For this review, take the finished solid that the model builds, in its own axes (mm). Coordinates: 2 decimals unless noted, no trailing zeros. Write each loop counter-clockwise with the first axis right and the second up, starting at its lowest first coordinate (ties: lowest second). Pieces come first, ordered by that corner, then holes. Notation, with made-up numbers: (60, 67) -> (80, 67) arc R37 ccw to (80, 104) -> close; hole circle Ø3 at (81.25, 66.25). An arc over 180 degrees is marked (long way). Put each result on its own line as item: value. Start each with the question number.
Item 1: To check wall thickness, follow L1, parallel to Z at x = -25, y = 3.2; L2, parallel to Z at x = -43.5, y = 0.3; L3, parallel to X at y = 1.55, z = 52. State the ranges of each line that lie inside material, in increasing order.
Item 2: Consider section C-C on x = -75. Give the boundary of the cut face in (y, z), and give its area (3 significant figures).
Item 3: Consider section B-B on z = -6. Give the boundary of the cut face in (x, y), and give its area (3 significant figures).
Item 4: Insertion check: P1, Ø10, axis at x = 44, z = 39.5, coming from the -Y side. The pin has a flat end and moves straight along its axis. Give the tip position at first contact, or say it passes through.
Item 5: The part is to be moulded in two halves that separate along Z. For faces 1 (the flat face through (-31, 0, -1)), 2 (the cylindrical face through (126.99, 2.03, -66.15)), 3 (the cylindrical face through (126.99, 2.03, 66.15)), 4 (the cylindrical face through (7.21, 2.03, 22.89)), say which applies: +Z half, -Z half, draft (parallel to the pull), parting line (faces both ways), or undercut.
Item 6: Consider section D-D on z = -20.5. Give the boundary of the cut face in (x, y), and give its area (3 significant figures).
Item 7: Consider section A-A on x = 0. Give the boundary of the cut face in (y, z), and give its area (3 significant figures).
```python
from build123d import *

# Parameters (mm, degrees)
SKETCH_1_W          = 260
SKETCH_1_H          = 138
SKETCH_1_R          = 1.35
EXTRUDE_1_DEPTH     = 4
SKETCH_3_R          = 24
SKETCH_3_R_2        = 1.65
CUT_EXTRUDE_1_DEPTH = 4
CUT_EXTRUDE_3_DEPTH = 4
FILLET_1_R          = 10


with BuildPart() as part:
    # 草图1 → 凸台-拉伸1 (new body)
    with BuildSketch(Plane(origin=(0, 0, 0), x_dir=(1, 0, 0), z_dir=(0, 1, 0))):
        Rectangle(SKETCH_1_W, SKETCH_1_H)
        with Locations(Location((-122, 64, 0), (0, 0, 270))):
            Circle(SKETCH_1_R, mode=Mode.SUBTRACT)
        with Locations(Location((122, 64, 0), (0, 0, 90))):
            Circle(SKETCH_1_R, mode=Mode.SUBTRACT)
        with Locations(Location((122, -64, 0), (0, 0, 270))):
            Circle(SKETCH_1_R, mode=Mode.SUBTRACT)
        with Locations(Location((-122, -64, 0), (0, 0, 90))):
            Circle(SKETCH_1_R, mode=Mode.SUBTRACT)
    extrude(amount=EXTRUDE_1_DEPTH)

    # 草图3 → 切除-拉伸1 (cut)
    with BuildSketch(Plane(origin=(0, 4, 0), x_dir=(1, 0, 0), z_dir=(0, 1, 0))):
        with Locations(Location((0, 0, 0), (0, 0, 270))):
            Circle(SKETCH_3_R)
        with Locations(Location((-29, 0, 0), (0, 0, 270))):
            Circle(SKETCH_3_R_2)
        with Locations(Location((14.5, 25.11473671, 0), (0, 0, 270))):
            Circle(SKETCH_3_R_2)
        with Locations(Location((14.5, -25.11473671, 0), (0, 0, 270))):
            Circle(SKETCH_3_R_2)
    extrude(amount=-CUT_EXTRUDE_1_DEPTH, mode=Mode.SUBTRACT)

    # 草图4 → 切除-拉伸3 (cut)
    with BuildSketch(Plane(origin=(0, 4, 0), x_dir=(1, 0, 0), z_dir=(0, 1, 0))):
        with BuildLine():
            Line((-111, 59), (-11, 59))
            ThreePointArc((-11, 59), (-10.292893219, 58.707106781), (-10, 58))
            Line((-10, 58), (-10, 45))
            ThreePointArc((-10, 45), (-10.292893219, 44.292893219), (-11, 44))
            Line((-11, 44), (-111, 44))
            ThreePointArc((-111, 44), (-111.707106781, 44.292893219), (-112, 45))
            Line((-112, 45), (-112, 58))
            ThreePointArc((-112, 58), (-111.707106781, 58.707106781), (-111, 59))
        make_face()
        with BuildLine():
            Line((-111, 24), (-40, 24))
            ThreePointArc((-40, 24), (-39.292893219, 23.707106781), (-39, 23))
            Line((-39, 23), (-39, 10))
            ThreePointArc((-39, 10), (-39.292893219, 9.292893219), (-40, 9))
            Line((-40, 9), (-111, 9))
            ThreePointArc((-111, 9), (-111.707106781, 9.292893219), (-112, 10))
            Line((-112, 10), (-112, 23))
            ThreePointArc((-112, 23), (-111.707106781, 23.707106781), (-111, 24))
        make_face()
        with BuildLine():
            Line((111, 9), (40, 9))
            ThreePointArc((40, 9), (39.292893219, 9.292893219), (39, 10))
            Line((39, 10), (39, 23))
            ThreePointArc((39, 23), (39.292893219, 23.707106781), (40, 24))
            Line((40, 24), (111, 24))
            ThreePointArc((111, 24), (111.707106781, 23.707106781), (112, 23))
            Line((112, 23), (112, 10))
            ThreePointArc((112, 10), (111.707106781, 9.292893219), (111, 9))
        make_face()
        with BuildLine():
            Line((111, 44), (11, 44))
            ThreePointArc((11, 44), (10.292893219, 44.292893219), (10, 45))
            Line((10, 45), (10, 58))
            ThreePointArc((10, 58), (10.292893219, 58.707106781), (11, 59))
            Line((11, 59), (111, 59))
            ThreePointArc((111, 59), (111.707106781, 58.707106781), (112, 58))
            Line((112, 58), (112, 45))
            ThreePointArc((112, 45), (111.707106781, 44.292893219), (111, 44))
        make_face()
        with BuildLine():
            Line((111, -9), (40, -9))
            ThreePointArc((40, -9), (39.292893219, -9.292893219), (39, -10))
            Line((39, -10), (39, -23))
            ThreePointArc((39, -23), (39.292893219, -23.707106781), (40, -24))
            Line((40, -24), (111, -24))
            ThreePointArc((111, -24), (111.707106781, -23.707106781), (112, -23))
            Line((112, -23), (112, -10))
            ThreePointArc((112, -10), (111.707106781, -9.292893219), (111, -9))
        make_face()
        with BuildLine():
            Line((-111, -9), (-40, -9))
            ThreePointArc((-40, -9), (-39.292893219, -9.292893219), (-39, -10))
            Line((-39, -10), (-39, -23))
            ThreePointArc((-39, -23), (-39.292893219, -23.707106781), (-40, -24))
            Line((-40, -24), (-111, -24))
            ThreePointArc((-111, -24), (-111.707106781, -23.707106781), (-112, -23))
            Line((-112, -23), (-112, -10))
            ThreePointArc((-112, -10), (-111.707106781, -9.292893219), (-111, -9))
        make_face()
        with BuildLine():
            Line((111, -44), (11, -44))
            ThreePointArc((11, -44), (10.292893219, -44.292893219), (10, -45))
            Line((10, -45), (10, -58))
            ThreePointArc((10, -58), (10.292893219, -58.707106781), (11, -59))
            Line((11, -59), (111, -59))
            ThreePointArc((111, -59), (111.707106781, -58.707106781), (112, -58))
            Line((112, -58), (112, -45))
            ThreePointArc((112, -45), (111.707106781, -44.292893219), (111, -44))
        make_face()
        with BuildLine():
            Line((-111, -44), (-11, -44))
            ThreePointArc((-11, -44), (-10.292893219, -44.292893219), (-10, -45))
            Line((-10, -45), (-10, -58))
            ThreePointArc((-10, -58), (-10.292893219, -58.707106781), (-11, -59))
            Line((-11, -59), (-111, -59))
            ThreePointArc((-111, -59), (-111.707106781, -58.707106781), (-112, -58))
            Line((-112, -58), (-112, -45))
            ThreePointArc((-112, -45), (-111.707106781, -44.292893219), (-111, -44))
        make_face()
    extrude(amount=-CUT_EXTRUDE_3_DEPTH, mode=Mode.SUBTRACT)

    # 圆角1
    fillet_1_edges = [part.edges().sort_by_distance(p)[0] for p in [
        (130, 2, 69),
        (-130, 2, 69),
        (-130, 2, -69),
        (130, 2, -69),
    ]]
    fillet(fillet_1_edges, radius=FILLET_1_R)


solid = part.part
```
Return value:
1. L1: -69 to -59, -44 to 44, 59 to 69
1. L2: -69 to -59, -44 to -24, -9 to 9, 24 to 44, 59 to 69
1. L3: -130 to -112, -10 to 10, 112 to 130
2. outline: (0, -69) -> (4, -69) -> (4, -59) -> (0, -59) -> close; (0, -44) -> (4, -44) -> (4, -24) -> (0, -24) -> close; (0, -9) -> (4, -9) -> (4, 9) -> (0, 9) -> close; (0, 24) -> (4, 24) -> (4, 44) -> (0, 44) -> close; (0, 59) -> (4, 59) -> (4, 69) -> (0, 69) -> close
2. area: 312 mm^2
3. outline: (-130, 0) -> (-23.24, 0) -> (-23.24, 4) -> (-130, 4) -> close; (23.24, 0) -> (130, 0) -> (130, 4) -> (23.24, 4) -> close
3. area: 854 mm^2
4. P1: y = 0
5. face 1: draft
5. face 2: -Z half
5. face 3: +Z half
5. face 4: undercut
6. outline: (-130, 0) -> (-112, 0) -> (-112, 4) -> (-130, 4) -> close; (-39, 0) -> (-12.48, 0) -> (-12.48, 4) -> (-39, 4) -> close; (12.48, 0) -> (39, 0) -> (39, 4) -> (12.48, 4) -> close; (112, 0) -> (130, 0) -> (130, 4) -> (112, 4) -> close
6. area: 356 mm^2
7. outline: (0, -69) -> (4, -69) -> (4, -24) -> (0, -24) -> close; (0, 24) -> (4, 24) -> (4, 69) -> (0, 69) -> close
7. area: 360 mm^2
